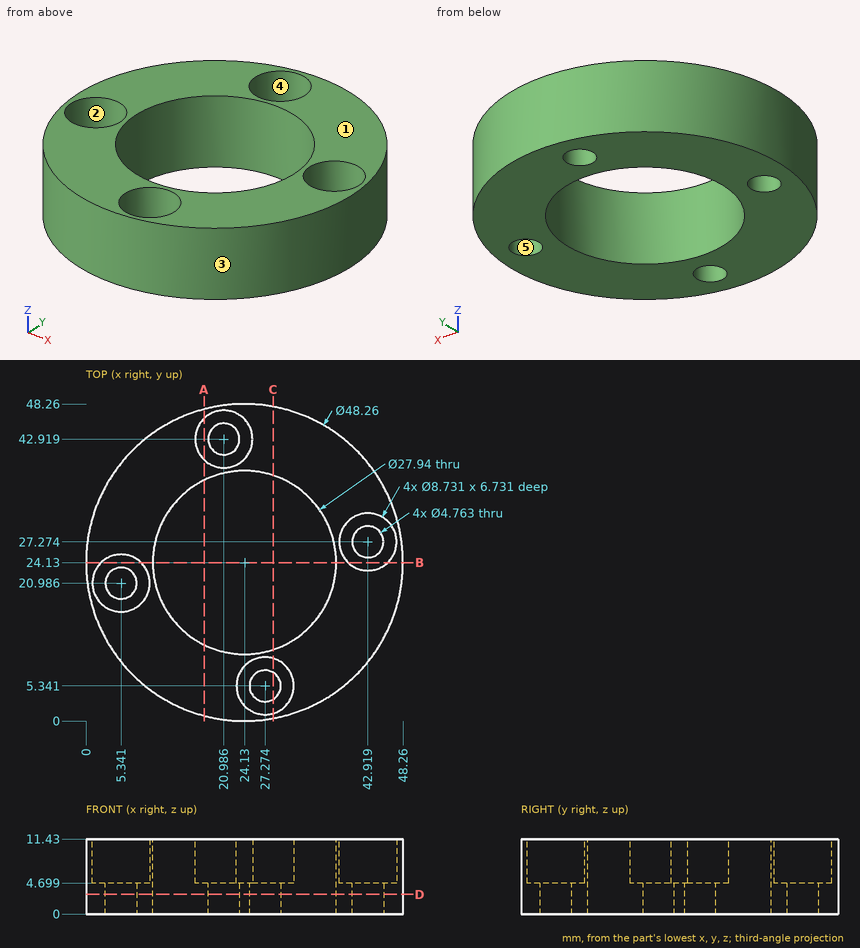
Print and shaded views of the part. All mm, measured from the part's lowest x, y and z. A direction names the side the tool comes from. Coordinates: 2 decimals unless noted, no trailing zeros. Loops run counter-clockwise (first coordinate to the right, second up) from the corner with the lowest first, then second, coordinate; pieces in that order, holes last. Notation, with made-up numbers: (-34.5, 30) - (6.5, 30) arc R7 ccw to (6.5, 38) - close; hole circle Ø11 at (64.25, 2). An arc over 180 degrees is marked (long way). Write item = value, one per line. Start each with the question number.
Item 1: Drop flat-ended pins along their axis: pin 1 Ø4.5 at (x, y) = (5.34, 20.99) entering from -Z; pin 2 Ø1.5 at (x, z) = (15.5, 9) entering from +Y; pin 3 Ø6 at (y, z) = (16, 3) entering from -X; pin 4 Ø3 at (x, z) = (42.5, 4) entering from -Y. Give the stop position or say it passes through.
Item 2: Pull direction X, two halves, no side cores. Call the marked faces 1, 2 and 3: +X half, -X half, draft (parallel to the pull), parting line (faces both ways), or undercut.
Item 3: Saw through at B-B, the plane y = 24.13. List the corners of the cut face in (x, z), then the cut area to 3 significant figures.
Item 4: Saw through at D-D, the plane z = 3. List the corners of the cut face in (x, y) (1 decimal).
Item 5: Saw through at A-A, the plane x = 18. List the corners of the cut face in (y, z), then the cut area to 3 significant figures.
Item 6: Saw through at C-C, the plane x = 28.5. List the corners of the cut face in (y, z).
Item 7: 3-axis set-ups, long thin cutter, end or side, ignore diameter. For the marked faces 4 and 5: which of +Z, -Z, +X, -X, +Y, -Y reach the whole face in a straight line?
Item 8: Wall check: probe 1 along X at (y, z) = (18, 6.25) (1 decimal); probe 2 along Y at (x, z) = (28, 0.75); probe 3 along X at (y, z) = (26.5, 1). Give the ranges that are in metal, low to high. Write a range as [from, to].
Answers:
q1.pin_1 = through
q1.pin_2 = 46.94
q1.pin_3 = 0.55
q1.pin_4 = 6.88
q2.face_1 = draft
q2.face_2 = undercut
q2.face_3 = parting line
q3.outline = (0, 0) - (10.16, 0) - (10.16, 11.43) - (8.37, 11.43) - (8.37, 4.7) - (2.31, 4.7) - (2.31, 11.43) - (0, 11.43) - close; (38.1, 0) - (48.26, 0) - (48.26, 11.43) - (45.95, 11.43) - (45.95, 4.7) - (39.89, 4.7) - (39.89, 11.43) - (38.1, 11.43) - close
q3.area = 151 mm2
q4.outline = circle Ø48.3 at (24.1, 24.1); hole circle Ø4.8 at (5.3, 21); hole circle Ø27.9 at (24.1, 24.1); hole circle Ø4.8 at (21, 42.9); hole circle Ø4.8 at (27.3, 5.3); hole circle Ø4.8 at (42.9, 27.3)
q5.outline = (0.79, 0) - (11.58, 0) - (11.58, 11.43) - (0.79, 11.43) - close; (36.68, 0) - (47.47, 0) - (47.47, 11.43) - (46.1, 11.43) - (46.1, 4.7) - (39.73, 4.7) - (39.73, 11.43) - (36.68, 11.43) - close
q5.area = 204 mm2
q6.outline = (0.4, 0) - (3.3, 0) - (3.3, 4.7) - (1.15, 4.7) - (1.15, 11.43) - (0.4, 11.43) - close; (7.38, 0) - (10.86, 0) - (10.86, 11.43) - (9.53, 11.43) - (9.53, 4.7) - (7.38, 4.7) - close; (37.4, 0) - (47.86, 0) - (47.86, 11.43) - (37.4, 11.43) - close
q7.face_4 = +Z
q7.face_5 = +Z, -Z
q8.probe_1 = [0.8, 2.2], [8.5, 11.6], [36.7, 47.5]
q8.probe_2 = [0.31, 3.07], [7.61, 10.71], [37.55, 47.95]
q8.probe_3 = [0.12, 10.36], [37.9, 40.67], [45.17, 48.14]
